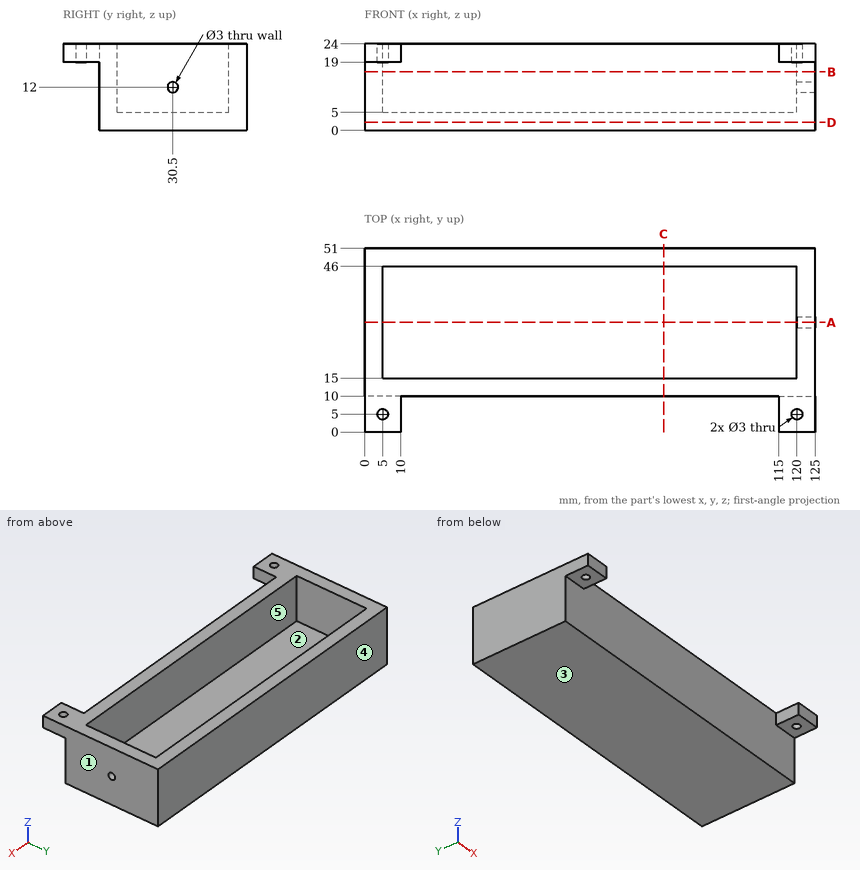
Check sheet for the drawn part. Datum: minimum x, y, z corner. Units: mm. A direction names the side the tool comes from. Give positions to 0.01 mm unless a question says otherwise; leave off trailing zeros. Order: outer loops, then holes, each group sorted by start corner. A loop starts at its lowest first (then second) coordinate and runs counter-clockwise, first axis right, second up. Notation, with made-up numbers: (87, 16.5) - (124, 16.5) arc R22 cw to (124, 36.5) - close; hole circle Ø3 at (78.25, 62.25). An arc over 180 degrees is marked (long way). Answer in a Markdown table with one row per item. Add a question column.
Q1. Gauge pin test, flat ends, axial feed: pin 1 (8 mm diameter, centred on x = 119, y = 3.5, fed in from -Z); pin 2 (1.5 mm diameter, centred on x = 37.5, z = 6.5, fed in from -Y); pin 3 (2.5 mm diameter, centred on x = 5, y = 5, fed in from +Z). Record the tip position at first contact, or that the pin passes through.
Q2. Cross-section at A-A, the plane y = 30.5. Enter the section's corners in (x, z), then the cut area to 3 significant figures.
Q3. Cross-section at B-B, the plane z = 16.25. Enter the section's corners in (x, y), then the cut area to 3 significant figures.
Q4. Cross-section at C-C, the plane x = 83. Enter the section's corners in (y, z).
Q5. Tool access check on the marked faces 4 and 5. Record the directions out of +Z, -Z, +X, -X, +Y, -Y that give a thin tool (end or side, any length) a straight path to the whole face; none if there is none.
Q6. Cross-section at D-D, the plane z = 2.25. Enter the section's corners in (x, y), then the cut area to 4 significant figures.
Q7. Material ranges on probe 1 along X at (y, z) = (43, 5.75); probe 2 along Y at (x, z) = (102, 13); probe 3 along Z at (x, y) = (84.5, 44), recorded low to high. Write a range as from..to.
Q8. Mould release check, pull along X, two halves, no side actions. Record for the marked faces 1, 2 and 3: pulls with the +X half, pulls with the -X half, needs draft (parallel to the pull), parting line crosses it, or undercut.
Check values:
| question | item | result |
|---|---|---|
| 1 | pin 1 | stops at z = 19 |
| 1 | pin 2 | stops at y = 10 |
| 1 | pin 3 | passes through |
| 2 | outline | (0, 0) - (125, 0) - (125, 10.5) - (120, 10.5) - (120, 5) - (5, 5) - (5, 24) - (0, 24) - close; (120, 13.5) - (125, 13.5) - (125, 24) - (120, 24) - close |
| 2 | area | 800 mm^2 |
| 3 | outline | (0, 10) - (125, 10) - (125, 51) - (0, 51) - close; hole (5, 15) - (120, 15) - (120, 46) - (5, 46) - close |
| 3 | area | 1,560 mm^2 |
| 4 | outline | (10, 0) - (51, 0) - (51, 24) - (46, 24) - (46, 5) - (15, 5) - (15, 24) - (10, 24) - close |
| 5 | face 4 | +Z, -Z, +X, -X, +Y |
| 5 | face 5 | +Z |
| 6 | outline | (0, 10) - (125, 10) - (125, 51) - (0, 51) - close |
| 6 | area | 5,125 mm^2 |
| 7 | probe 1 | x = 0..5, 120..125 |
| 7 | probe 2 | y = 10..15, 46..51 |
| 7 | probe 3 | z = 0..5 |
| 8 | face 1 | pulls with the +X half |
| 8 | face 2 | undercut |
| 8 | face 3 | needs draft |
